Input: dimensioned drawing with shaded views. Units: mm. Origin: part minimum x, y, z. A direction names the side the tool comes from. Coordinates: 2 decimals unless noted, no trailing zeros. Loops run counter-clockwise (first coordinate to the right, second up) from the corner with the lowest first, then second, coordinate; pieces in that order, holes last. Notation, with made-up numbers: (26, 73) -> (76, 73) arc R10 cw to (76, 88) -> close; hole circle Ø3 at (12.25, 15). An arc over 180 degrees is marked (long way). Answer as CSV lines item,"result".
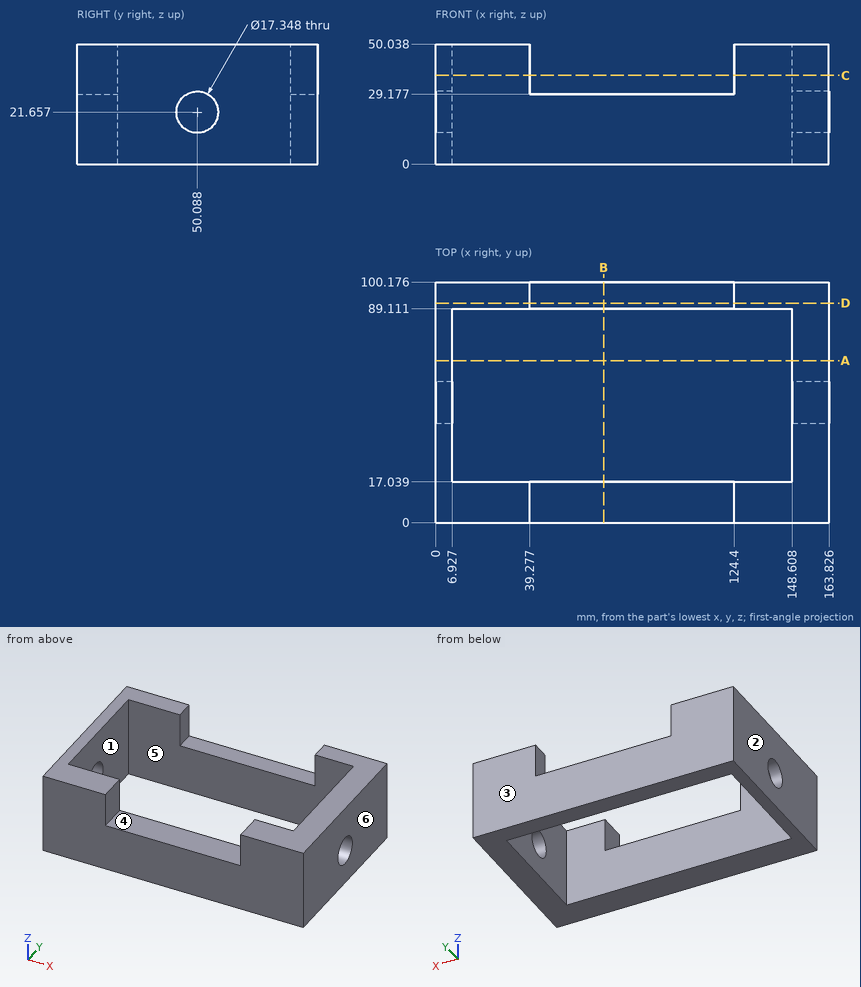
(1) Cut plane B-B (x = 70). Return the cut outline in (y, z).
Computed values:
outline,"(0, 0) -> (17.04, 0) -> (17.04, 29.18) -> (0, 29.18) -> close; (89.11, 0) -> (100.18, 0) -> (100.18, 29.18) -> (89.11, 29.18) -> close"
(2) Pin query (flat end, axial travel): pin 1 Ø5 at (x, y) = (73, 5) entering from +Z; pin 2 Ø4 at (x, y) = (146.5, 75.5) entering from +Z. Return the tip coordinate at first contact, or that it passes through.
Computed values:
pin 1,"z = 29.18"
pin 2,"through"
(3) Draft query along X for the marked faces 1, 2, 3 and 4. Return one class per face: released by +X, released by -X, zero draft, split by the parting line, or undercut.
Computed values:
face 1,"undercut"
face 2,"released by -X"
face 3,"zero draft"
face 4,"undercut"
(4) Cut plane A-A (y = 67.5). Return the cut outline in (x, z) (1 decimal).
Computed values:
outline,"(0, 0) -> (6.9, 0) -> (6.9, 50) -> (0, 50) -> close; (148.6, 0) -> (163.8, 0) -> (163.8, 50) -> (148.6, 50) -> close"
(5) Access query for the marked faces 5 and 6. Directions: +Z, -Z, +X, -X, +Y, -Y. A direction counts if a zero-diameter tool reaches every point of the face in a straight line with its end or side. Return the directions, or none.
Computed values:
face 5,"+Z, -Z"
face 6,"+Z, -Z, +X, +Y, -Y"
(6) Cut plane D-D (y = 91.5). Return the cut outline in (x, z) (1 decimal), then the cut area to 3 significant figures.
Computed values:
outline,"(0, 0) -> (163.8, 0) -> (163.8, 50) -> (124.4, 50) -> (124.4, 29.2) -> (39.3, 29.2) -> (39.3, 50) -> (0, 50) -> close"
area,"6,420 mm^2"
(7) Cut plane C-C (z = 37). Return the cut outline in (x, y) (1 decimal), then the cut area to 3 significant figures.
Computed values:
outline,"(0, 0) -> (39.3, 0) -> (39.3, 17) -> (6.9, 17) -> (6.9, 89.1) -> (39.3, 89.1) -> (39.3, 100.2) -> (0, 100.2) -> close; (124.4, 0) -> (163.8, 0) -> (163.8, 100.2) -> (124.4, 100.2) -> (124.4, 89.1) -> (148.6, 89.1) -> (148.6, 17) -> (124.4, 17) -> close"
area,"3,810 mm^2"
(8) Material intervals for L1, parallel to Y at x = 10, z = 23.5; L2, parallel to X at y = 69.5, z = 35.5 (1 decimal); L3, parallel to Z at x = 61.5, y = 12.5, sorted ascending. Write a range as [from, to].
Computed values:
L1,"[0, 17.04], [89.11, 100.18]"
L2,"[0, 6.9], [148.6, 163.8]"
L3,"[0, 29.18]"
